Part model, mm, in its own coordinate system. Face numbers are marked on the shaded views. A direction names the side the tool comes from. Give positions to 0.01 mm unless a question says otherwise; leave off trailing zeros. Order: outer loops, then holes, each group sorted by start corner. A loop starts at its lowest first (then second) coordinate and runs counter-clockwise, first axis right, second up. Notation, with made-up numbers: M 66,17 L 122,17 A6 ccw 122,25 Z; hole C -21,52 d6. An arc over 180 degrees is marked long. One line per question, with ' | ' between items.
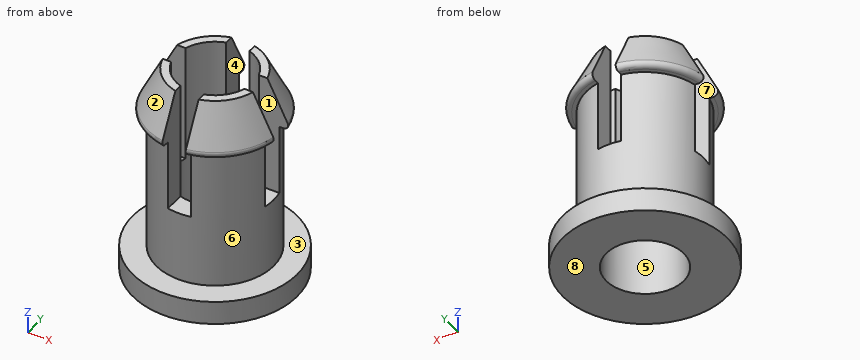
```python
from build123d import *

# Parameters (mm, degrees)
BOX002_W               = 1
BOX002_H               = 10
BOX002_DEPTH           = 10
BOX003_W               = 1
BOX003_H               = 10
BOX003_DEPTH           = 10
BOX003_PLACEMENT_ANGLE = 90
CYLINDER013_R          = 1.65
CYLINDER013_DEPTH      = 14
CYLINDER011_R          = 2.5
CYLINDER011_DEPTH      = 7.5
CYLINDER012_R          = 3.5
CYLINDER012_DEPTH      = 1
FILLET002_R            = 0.2


with BuildPart() as cube002:
    # Box002 → Box002 (new body)
    with BuildSketch(Plane(origin=(-0.5, -5, 0), x_dir=(1, 0, 0), z_dir=(0, 0, 1))):
        with Locations((0.5, 5)):
            Rectangle(BOX002_W, BOX002_H)
    extrude(amount=BOX002_DEPTH)


with BuildPart() as fusion011:
    # Box003 → Box003 (new body)
    with BuildSketch(Plane.XY):
        with Locations((0.5, 5)):
            Rectangle(BOX003_W, BOX003_H)
    extrude(amount=BOX003_DEPTH)


with BuildPart() as fusion011_1:
    # Box003 placement: moved
    add(fusion011.part.moved(Location((5, -0.5, 0))).rotate(Axis((5, -0.5, 0), (0, 0, 1)), BOX003_PLACEMENT_ANGLE))

    # Fusion011: union Cube002
    add(cube002.part)


with BuildPart() as fusion011_2:
    # Fusion011 placement: moved
    add(fusion011_1.part.moved(Location((0, 0, 4))))


with BuildPart() as cylinder013:
    # Cylinder013 → Cylinder013 (new body)
    with BuildSketch(Plane.XY.offset(-1)):
        Circle(CYLINDER013_R)
    extrude(amount=CYLINDER013_DEPTH)


with BuildPart() as cylinder011:
    # Cylinder011 → Cylinder011 (new body)
    with BuildSketch(Plane.XY):
        Circle(CYLINDER011_R)
    extrude(amount=CYLINDER011_DEPTH)


with BuildPart() as cylinder012:
    # Cylinder012 → Cylinder012 (new body)
    with BuildSketch(Plane.XY):
        Circle(CYLINDER012_R)
    extrude(amount=CYLINDER012_DEPTH)


with BuildPart() as cut008:
    # Cone → Cone (revolve)
    with BuildSketch(Plane(origin=(0, 0, 7), x_dir=(1, 0, 0), z_dir=(0, -1, 0))):
        Polygon((0, 0), (3, 0), (2, 2), (0, 2), align=None)
    revolve(axis=Axis((0, 0, 7), (0, 0, 1)))

    # Fillet002
    fillet002_edges = [cut008.edges().sort_by_distance(p)[0] for p in [
        (-3, 0, 7),
    ]]
    fillet(fillet002_edges, radius=FILLET002_R)

    # Fusion012: union Cylinder011, Cylinder012
    add(cylinder011.part)
    add(cylinder012.part)

    # Cut007: cut Cylinder013
    add(cylinder013.part, mode=Mode.SUBTRACT)

    # Cut008: cut Fusion011
    add(fusion011_2.part, mode=Mode.SUBTRACT)


solid = cut008.part
```
1. Tool access for the marked faces 1, 2, 3, 4 and 5: list every direction of +Z, -Z, +X, -X, +Y, -Y with a clear straight run to the whole face (end or side of a thin tool).
Worked out:
face 1: +Z, +X, -X | face 2: +Z, -X, -Y | face 3: none | face 4: +Z, +Y, -Y | face 5: +Z, -Z
2. Probe L1, parallel to X at y = 0, z = 2; L2, parallel to Z at x = -2, y = -2.5. List the from-to ranges inside material, lowest first. Write a range as from..to.
Worked out:
L1: x = -2.5..-1.65, 1.65..2.5 | L2: z = 0..1
3. Slice it at A-A on x = 0. Give the cut face in (y, z).
Worked out:
outline: M -3.5,0 L -1.65,0 L -1.65,4 L -2.5,4 L -2.5,1 L -3.5,1 Z; M 1.65,0 L 3.5,0 L 3.5,1 L 2.5,1 L 2.5,4 L 1.65,4 Z
4. Slice it at C-C on z = 5. Give the cut face in (x, y).
Worked out:
outline: M -2.45,-0.5 A2.5 ccw -0.5,-2.45 L -0.5,-1.57 A1.65 cw -1.57,-0.5 Z; M -2.45,0.5 L -1.57,0.5 A1.65 cw -0.5,1.57 L -0.5,2.45 A2.5 ccw Z; M 0.5,-2.45 A2.5 ccw 2.45,-0.5 L 1.57,-0.5 A1.65 cw 0.5,-1.57 Z; M 0.5,1.57 A1.65 cw 1.57,0.5 L 2.45,0.5 A2.5 ccw 0.5,2.45 Z
5. Mould opens along Z. For the marked faces 6, 7 and 8 say: released by +Z, released by -Z, zero draft, split by the parting line, or undercut.
Worked out:
face 6: undercut | face 7: zero draft | face 8: released by -Z
6. Drop flat-ended pins along their axis: pin 1 (4 mm diameter, centred on x = -2.5, z = 2, fed in from +Y); pin 2 (2 mm diameter, centred on y = 1, z = 3, fed in from +X); pin 3 (1.4 mm diameter, centred on y = 2, z = 6.5, fed in from +X). Give the stop position or say it passes through.
Worked out:
pin 1: stops at y = 3.41 | pin 2: stops at x = 2.5 | pin 3: stops at x = 2.34
7. Slice it at D-D on z = 1.5. Give the cut face in (x, y).
Worked out:
outline: C 0,0 d5; hole C 0,0 d3.3
